Here's how the part is built. I have some questions about the finished solid (model axes, mm). A direction names the side the tool comes from. Give positions to 0.01 mm unless a question says otherwise; leave off trailing zeros. Loops run counter-clockwise (first coordinate to the right, second up) from the corner with the lowest first, then second, coordinate; pieces in that order, holes last.
Q1. I'm going to push flat-ended pins straight in: P1, Ø4, axis at x = -95.5, y = 3, coming from the +Z side; P2, Ø1.5, axis at x = -75.5, z = -0.5, coming from the +Y side; P3, Ø8, axis at x = -111.5, z = 2.5, coming from the +Y side. Where does each tip first touch, or does it pass through?
Q2. I need wall thicknesses on probe 1 along X at (y, z) = (-30.5, -9.5); probe 2 along Z at (x, y) = (5, -115.5); probe 3 along Y at (x, z) = (6, -2). Which ranges of each line are inside material? Lowest first, please.
Q3. Thinking about a two-plate mould opening in Y: for faces 1 (the face through (110.673, -28.794, -6.261)), 2 (the face through (32, 2, 0)), 3 (the face through (-120.94, -92.73, -6.26)), which applies, pulls with the +Y half, pulls with the -Y half, needs draft (parallel to the pull), parting line crosses it, or undercut?
Q4. Suppose I cut it at C-C (y = 32). List the corners of the cut face in (x, z) for me, and give its area (3 significant figures).
Q5. Suppose I cut it at A-A (y = 0). List the corners of the cut face in (x, z) for me, and give its area (3 significant figures).
Q6. For faces 4 (the face through (33.13, 110.48, -6.26)), 5 (the face through (4.13, 18.597, 12.611)), which set-ups out of +Z, -Z, +X, -X, +Y, -Y let a thin tool reach every point of the face, with its end or its side?
Q7. Suppose I cut it at D-D (z = -6). Count the separate pieces of the cut face and the enclosed holes in it, and give its area (3 significant figures).
```python
from build123d import *

# Parameters (mm, degrees)
SKETCH2_R           = 152.4
SKETCH2_R_2         = 12.7
BOSS_EXTRUDE1_DEPTH = 12.7
SKETCH3_R           = 6.35
CUT_EXTRUDE1_DEPTH  = 216.9
CRVPATTERN1_COUNT   = 12
SKETCH5_R           = 19.05
BOSS_EXTRUDE2_DEPTH = 19.05
SKETCH6_R           = 25.4
BOSS_EXTRUDE3_DEPTH = 6.35
SKETCH8_R           = 12.7
CUT_EXTRUDE2_DEPTH  = 218.85220334


with BuildPart() as part:
    # Sketch2 → Boss-Extrude1 (new body)
    with BuildSketch(Plane.XY):
        Circle(SKETCH2_R)
        Circle(SKETCH2_R_2, mode=Mode.SUBTRACT)
    extrude(amount=-BOSS_EXTRUDE1_DEPTH)

    # Sketch3 → Cut-Extrude1 (cut, through all)
    with BuildSketch(Plane.XY):
        with Locations((85.31243315, 85.31243315)):
            Circle(SKETCH3_R)
    cut_extrude1 = extrude(amount=-CUT_EXTRUDE1_DEPTH, mode=Mode.SUBTRACT)

    # CrvPattern1: Cut-Extrude1 ×12 about axis
    crvpattern1_axis = Axis((0, 0, 0), (0, 0, 1))
    for i in range(1, CRVPATTERN1_COUNT):
        add(cut_extrude1.rotate(crvpattern1_axis, i * 360 / CRVPATTERN1_COUNT), mode=Mode.SUBTRACT)

    # Sketch5 → Boss-Extrude2 (add)
    with BuildSketch(Plane.XY):
        with Locations(Location((0, 0, 0), (0, 0, 180))):
            Circle(SKETCH5_R)
    extrude(amount=BOSS_EXTRUDE2_DEPTH)

    # Sketch6 → Boss-Extrude3 (add)
    with BuildSketch(Plane.XY):
        Circle(SKETCH6_R)
    extrude(amount=BOSS_EXTRUDE3_DEPTH)

    # Sketch8 → Cut-Extrude2 (cut, through all)
    with BuildSketch(Plane(origin=(0, 0, -12.7), x_dir=(-1, 0, 0), z_dir=(0, 0, -1))):
        with Locations(Location((0, 0, 0), (0, 0, 180))):
            Circle(SKETCH8_R)
    extrude(amount=-CUT_EXTRUDE2_DEPTH, mode=Mode.SUBTRACT)


solid = part.part
```
Solutions:
1. P1: stops at z = 0
1. P2: stops at y = 132.81
1. P3: stops at y = 107.15
2. probe 1: x = -149.32 to -122.85, -110.23 to 110.23, 122.85 to 149.32
2. probe 2: z = -12.7 to 0
2. probe 3: y = -152.28 to -11.19, 11.19 to 152.28
3. face 1: undercut
3. face 2: needs draft
3. face 3: parting line crosses it
4. outline: (-149, -12.7) - (-122.84, -12.7) - (-122.84, 0) - (-149, 0) - close; (-110.24, -12.7) - (110.24, -12.7) - (110.24, 0) - (-110.24, 0) - close; (122.84, -12.7) - (149, -12.7) - (149, 0) - (122.84, 0) - close
4. area: 3,460 mm2
5. outline: (-152.4, -12.7) - (-12.7, -12.7) - (-12.7, 19.05) - (-19.05, 19.05) - (-19.05, 6.35) - (-25.4, 6.35) - (-25.4, 0) - (-152.4, 0) - close; (12.7, -12.7) - (152.4, -12.7) - (152.4, 0) - (25.4, 0) - (25.4, 6.35) - (19.05, 6.35) - (19.05, 19.05) - (12.7, 19.05) - close
5. area: 3,870 mm2
6. face 4: +Z, -Z
6. face 5: +Z
7. separate pieces: 1
7. enclosed holes: 13
7. area: 70,900 mm2
